from build123d import *

# Parameters (mm, degrees)
SKETCH1_R           = 35
SKETCH1_R_2         = 30
BOSS_EXTRUDE1_DEPTH = 10
BOSS_EXTRUDE2_START = 3
BOSS_EXTRUDE2_DEPTH = 3
SKETCH3_W           = 10
SKETCH3_H           = 102
BOSS_EXTRUDE3_DEPTH = 3
SKETCH6_W           = 2.1
SKETCH6_H           = 95.310889132
CIRPATTERN1_COUNT   = 3
CUT_EXTRUDE1_REACH  = 137


with BuildPart() as part:
    # Sketch1 → Boss-Extrude1 (new, symmetric)
    with BuildSketch(Plane.XY):
        Circle(SKETCH1_R)
        Circle(SKETCH1_R_2, mode=Mode.SUBTRACT)
    extrude(amount=BOSS_EXTRUDE1_DEPTH, both=True)

    # Sketch2 → Boss-Extrude2 (add)
    with BuildSketch(Plane.XY.offset(BOSS_EXTRUDE2_START)):
        with BuildLine():
            Line((-21, 130), (21, 130))
            Line((21, 130), (21, 28))
            ThreePointArc((21, 28), (0, 35), (-21, 28))
            Line((-21, 28), (-21, 130))
        make_face()
    extrude(amount=-BOSS_EXTRUDE2_DEPTH)

    # Sketch3 → Boss-Extrude3 (add)
    with BuildSketch(Plane.ZY.offset(21)):
        with Locations((5, 79)):
            Rectangle(SKETCH3_W, SKETCH3_H)
    boss_extrude3 = extrude(amount=-BOSS_EXTRUDE3_DEPTH)

    # Mirror1: Boss-Extrude3 across plane
    add(boss_extrude3.mirror(Plane(origin=(0, 0, 0), x_dir=(0, 0, 1), z_dir=(1, 0, 0))))

    # Sketch6 → M5x0.8 Tapped Hole1 (revolve, cut)
    with BuildSketch(Plane(origin=(0, 0, -2), x_dir=(0, 0, 1), z_dir=(1, 0, 0))):
        with Locations((1.05, 47.655444566)):
            Rectangle(SKETCH6_W, SKETCH6_H)
    m5x0_8_tapped_hole1 = revolve(axis=Axis((0, 6.35, -2), (0, -1, 0)), mode=Mode.SUBTRACT)

    # CirPattern1: M5x0.8 Tapped Hole1 ×3 about axis
    cirpattern1_axis = Axis((0, 0, 10), (0, 0, -1))
    for i in range(1, CIRPATTERN1_COUNT):
        add(m5x0_8_tapped_hole1.rotate(cirpattern1_axis, i * 360 / CIRPATTERN1_COUNT), mode=Mode.SUBTRACT)

    # Sketch7 → Cut-Extrude1 (cut, up to next)
    with BuildSketch(Plane(origin=(0, 0, 0), x_dir=(-1, 0, 0), z_dir=(0, 0, -1)), mode=Mode.PRIVATE) as cut_extrude1_sk1:
        with BuildLine():
            Line((2.5, 120), (2.5, 60))
            ThreePointArc((2.5, 60), (0, 57.5), (-2.5, 60))
            Line((-2.5, 60), (-2.5, 120))
            ThreePointArc((-2.5, 120), (0, 122.5), (2.5, 120))
        make_face()
    cut_extrude1_tool1 = extrude(cut_extrude1_sk1.sketch, amount=-CUT_EXTRUDE1_REACH, mode=Mode.PRIVATE) & part.part
    add(cut_extrude1_tool1.solids().sort_by_distance((0, 90, 0))[0], mode=Mode.SUBTRACT)


solid = part.part
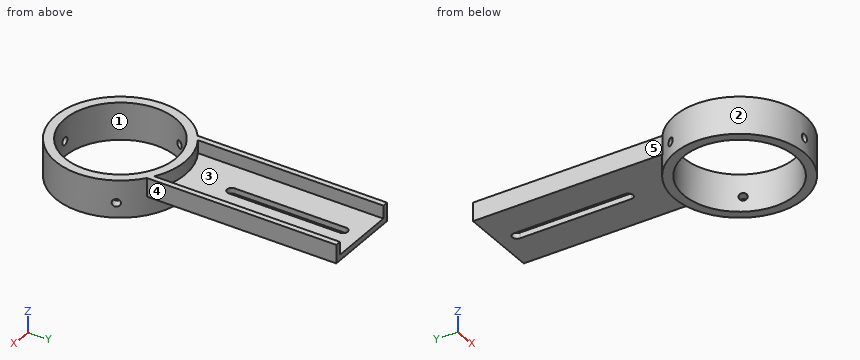
Part model, mm, in its own coordinate system. Face numbers are marked on the shaded views. A direction names the side the tool comes from. Round coordinates to 2 decimals unless told otherwise and drop trailing zeros. Loops run counter-clockwise (first coordinate to the right, second up) from the corner with the lowest first, then second, coordinate; pieces in that order, holes last. Notation, with made-up numbers: (-38.75, -34.5) - (5.25, -34.5) arc R7 cw to (5.25, -22.5) - close; hole circle Ø8 at (78.5, 87.25). An arc over 180 degrees is marked (long way). Answer as a JSON object with one key per item and string values.
Item 1: Pin check, flat tips, straight feed: pin 1 (3.5 mm diameter, centred on x = 0, z = -2, fed in from -Y); pin 2 (3 mm diameter, centred on y = 94.5, z = 5.5, fed in from -X); pin 3 (8 mm diameter, centred on x = 15, z = -4.5, fed in from +Y). Stop position of each tip, or through.
Output:
{"pin 1": "y = 29.95", "pin 2": "x = -21", "pin 3": "y = 33.23"}
Item 2: Pull direction Y, two halves, no side cores. Call the marked faces 1, 2 and 3: pulls with the +Y half, pulls with the -Y half, needs draft (parallel to the pull), parting line crosses it, or undercut.
Output:
{"face 1": "undercut", "face 2": "parting line crosses it", "face 3": "needs draft"}
Item 3: Band-saw the part on B-B on x = 0. List the corners of the cut face in (y, z).
Output:
{"outline": "(-35, -10) - (-30, -10) - (-30, -4.1) - (-35, -4.1) - close; (-35, 0.1) - (-30, 0.1) - (-30, 10) - (-35, 10) - close; (30, -10) - (35, -10) - (35, 0) - (57.5, 0) - (57.5, 3) - (35, 3) - (35, 10) - (30, 10) - close; (122.5, 0) - (130, 0) - (130, 3) - (122.5, 3) - close"}
Item 4: Wall check: L1, parallel to Y at x = 0, z = 2; L2, parallel to Z at x = 0, y = -33.6; L3, parallel to X at y = 96.5, z = 3.5. Give the ranges that are in metal, low to high.
Output:
{"L1": "-35 to -30, 30 to 57.5, 122.5 to 130", "L2": "-10 to -4.1, 0.1 to 10", "L3": "-21 to -18, 18 to 21"}
Item 5: Band-saw the part on A-A on z = 6.25. List the corners of the cut face in (x, y), plus the area to 3 significant figures.
Output:
{"outline": "(-21, 28) arc R35 ccw (long way) to (21, 28) - (21, 130) - (18, 130) - (18, 30.02) arc R35 ccw to (-18, 30.02) - (-18, 130) - (-21, 130) - close; hole circle Ø60 at (0, 0)", "area": "1,630 mm2"}
Item 6: Band-saw the part on C-C on y = 79. List the corners of the cut face in (x, z), plus the area to 3 significant figures.
Output:
{"outline": "(-21, 0) - (-2.5, 0) - (-2.5, 3) - (-18, 3) - (-18, 10) - (-21, 10) - close; (2.5, 0) - (21, 0) - (21, 10) - (18, 10) - (18, 3) - (2.5, 3) - close", "area": "153 mm2"}
Item 7: Tool access for the marked faces 4 and 5: list every direction of +Z, -Z, +X, -X, +Y, -Y with a clear straight run to the whole face (end or side of a thin tool).
Output:
{"face 4": "+Z, -Z, +X, +Y", "face 5": "+Z, -Z, -X, +Y"}
Item 8: Band-saw the part on D-D on x = 16. List the corners of the cut face in (y, z), plus the area to 3 significant figures.
Output:
{"outline": "(-31.13, -10) - (-25.38, -10) - (-25.38, 10) - (-31.13, 10) - close; (25.38, -10) - (31.13, -10) - (31.13, 0) - (130, 0) - (130, 3) - (31.13, 3) - (31.13, 10) - (25.38, 10) - close", "area": "527 mm2"}
